Can you work these out from the drawing? Everything is in mm from the part's minimum corner. Coordinates: 2 decimals unless noted, no trailing zeros. Order: outer loops, then holes, each group sorted by start corner. A loop starts at its lowest first (then second) coordinate and runs counter-clockwise, first axis right, second up. Notation, with made-up numbers: (75, 0.25) - (124, 0.25) arc R33 ccw to (124, 35.25) - close; hole circle Ø10 at (-33, -11.75). An arc over 180 degrees is marked (long way). Answer as CSV lines item,"result". Start each with the question number.
Item 1: Imagine slicing it at B-B on x = 9. List the corners of the cut face in (y, z) for me.
Item 2: Imagine slicing it at C-C on z = 1.25. List the corners of the cut face in (x, y) for me, and give its area (3 significant figures).
Item 3: Imagine slicing it at A-A on y = 12.51. List the corners of the cut face in (x, z) for me, and give its area (3 significant figures).
Item 4: Imagine slicing it at D-D on x = 46. List the corners of the cut face in (y, z) for me.
Item 5: I'm going to push a flat-ended pin straight in: pin 1 (0.8 mm diameter, centred on y = 8, z = 1, fed in from -X). Where does the tip first touch, or does it pass through?
Item 6: I need wall thicknesses on line 1 (X direction, y = 12.5, z = 1.35); line 2 (Y direction, x = 46.5, z = 0.75); line 3 (X direction, y = 16.5, z = 0.3). Which ranges of each line are inside material? Lowest first, please.
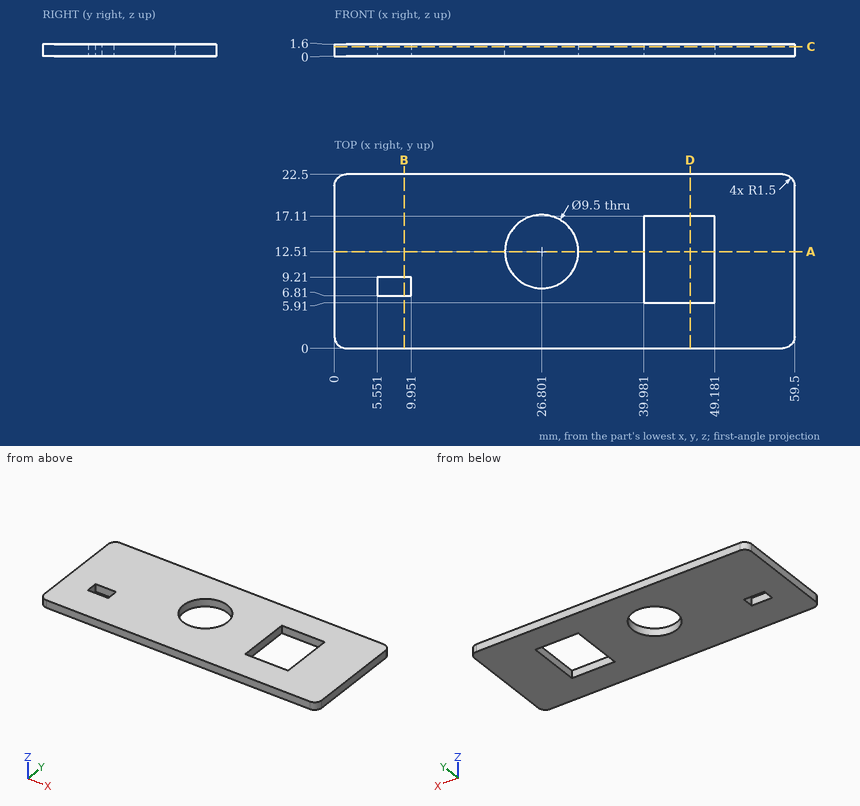
Responses:
1,outline,"(0, 0) - (6.81, 0) - (6.81, 1.6) - (0, 1.6) - close; (9.21, 0) - (22.5, 0) - (22.5, 1.6) - (9.21, 1.6) - close"
2,outline,"(0, 1.5) arc R1.5 ccw to (1.5, 0) - (58, 0) arc R1.5 ccw to (59.5, 1.5) - (59.5, 21) arc R1.5 ccw to (58, 22.5) - (1.5, 22.5) arc R1.5 ccw to (0, 21) - close; hole (5.55, 6.81) - (9.95, 6.81) - (9.95, 9.21) - (5.55, 9.21) - close; hole circle Ø9.5 at (26.8, 12.51); hole (39.98, 5.91) - (49.18, 5.91) - (49.18, 17.11) - (39.98, 17.11) - close"
2,area,"1,150 mm^2"
3,outline,"(0, 0) - (22.05, 0) - (22.05, 1.6) - (0, 1.6) - close; (31.55, 0) - (39.98, 0) - (39.98, 1.6) - (31.55, 1.6) - close; (49.18, 0) - (59.5, 0) - (59.5, 1.6) - (49.18, 1.6) - close"
3,area,"65.3 mm^2"
4,outline,"(0, 0) - (5.91, 0) - (5.91, 1.6) - (0, 1.6) - close; (17.11, 0) - (22.5, 0) - (22.5, 1.6) - (17.11, 1.6) - close"
5,pin 1,"stops at x = 0"
6,line 1,"x = 0 to 22.05, 31.55 to 39.98, 49.18 to 59.5"
6,line 2,"y = 0 to 5.91, 17.11 to 22.5"
6,line 3,"x = 0 to 24.22, 29.38 to 39.98, 49.18 to 59.5"
